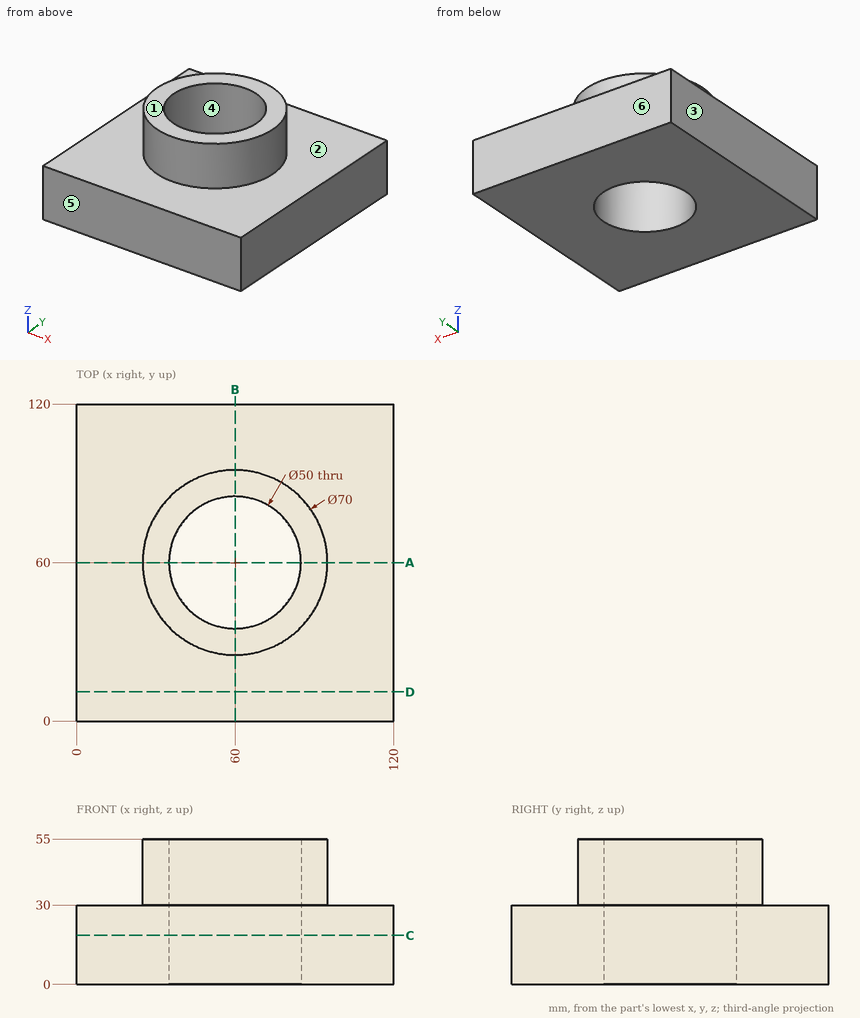
The drawing under review shows one solid part. Ordinate dimensions are in mm from its lowest x, y, z. A direction names the side the tool comes from. Coordinates: 2 decimals unless noted, no trailing zeros. Loops run counter-clockwise (first coordinate to the right, second up) from the corner with the lowest first, then second, coordinate; pieces in that order, holes last. Notation, with made-up numbers: (57, -25.75) - (80, -25.75) arc R10 cw to (80, -11.75) - close; hole circle Ø9 at (85.25, 21). An arc over 180 degrees is marked (long way). Return JSON: item names as keys, results as strings.
Item 1: Insertion check: pin 1 (8 mm diameter, centred on x = 43, z = 46, fed in from -Y); pin 2 (6 mm diameter, centred on y = 51.5, z = 48.5, fed in from -X); pin 3 (2 mm diameter, centred on x = 32, z = 35, fed in from -Y). Each pin has a flat end and moves straight along its axis. Give the tip position at first contact, or say it passes through.
Determined:
{"pin 1": "stops at y = 27.5", "pin 2": "stops at x = 25.43", "pin 3": "stops at y = 37.73"}
Item 2: For line 1 (X direction, y = 59.5, z = 35.5) (3 decimals); line 2 (Y direction, x = 60, z = 21); line 3 (Z direction, x = 104, y = 51.5), list the stretches that pass through material, from the lowest coordinate up.
Determined:
{"line 1": "x = 25.004 to 35.005, 84.995 to 94.996", "line 2": "y = 0 to 35, 85 to 120", "line 3": "z = 0 to 30"}
Item 3: For the marked faces 1 and 2, list the 3-axis set-ups (+Z, -Z, +X, -X, +Y, -Y) from which the entire face can be reached by the end or side of a thin tool; tool diameter is ignored.
Determined:
{"face 1": "+Z, +X, -X, +Y, -Y", "face 2": "+Z"}
Item 4: Take a section at D-D (y = 11). Give the boundary of the cut face in (x, z), then the cut area to 3 significant figures.
Determined:
{"outline": "(0, 0) - (120, 0) - (120, 30) - (0, 30) - close", "area": "3,600 mm2"}
Item 5: Take a section at C-C (z = 18.5). Give the boundary of the cut face in (x, y).
Determined:
{"outline": "(0, 0) - (120, 0) - (120, 120) - (0, 120) - close; hole circle Ø50 at (60, 60)"}
Item 6: Mouldability with a two-part tool opening along Y and no side actions: class the marked faces 3, 4, 5 and 6 as pulls with the +Y half, pulls with the -Y half, needs draft (parallel to the pull), parting line crosses it, or undercut.
Determined:
{"face 3": "needs draft", "face 4": "undercut", "face 5": "pulls with the -Y half", "face 6": "pulls with the +Y half"}
Item 7: Take a section at A-A (y = 60). Give the boundary of the cut face in (x, z), then the cut area to 3 significant figures.
Determined:
{"outline": "(0, 0) - (35, 0) - (35, 55) - (25, 55) - (25, 30) - (0, 30) - close; (85, 0) - (120, 0) - (120, 30) - (95, 30) - (95, 55) - (85, 55) - close", "area": "2,600 mm2"}
